from build123d import *

# Parameters (mm, degrees)
EXTRUDE_1_DEPTH = 20
SKETCH_2_R      = 4
EXTRUDE_2_DEPTH = 5
SKETCH_3_W      = 6
SKETCH_3_H      = 6
EXTRUDE_3_DEPTH = 15


with BuildPart() as part:
    # 草图1 → 凸台-拉伸1 (new body)
    with BuildSketch(Plane.XY):
        with BuildLine():
            Line((0, 10), (50, 10))
            ThreePointArc((50, 10), (60, 0), (50, -10))
            Line((50, -10), (0, -10))
            ThreePointArc((0, -10), (-10, 0), (0, 10))
        make_face()
    extrude(amount=EXTRUDE_1_DEPTH)

    # 草图2 → 凸台-拉伸2 (add)
    with BuildSketch(Plane.XY.offset(20)):
        with Locations((50, 0)):
            Circle(SKETCH_2_R)
    extrude(amount=EXTRUDE_2_DEPTH)

    # 草图3 → 凸台-拉伸3 (add)
    with BuildSketch(Plane(origin=(0, 0, 0), x_dir=(-1, 0, 0), z_dir=(0, 0, -1))):
        Rectangle(SKETCH_3_W, SKETCH_3_H)
    extrude(amount=EXTRUDE_3_DEPTH)


solid = part.part
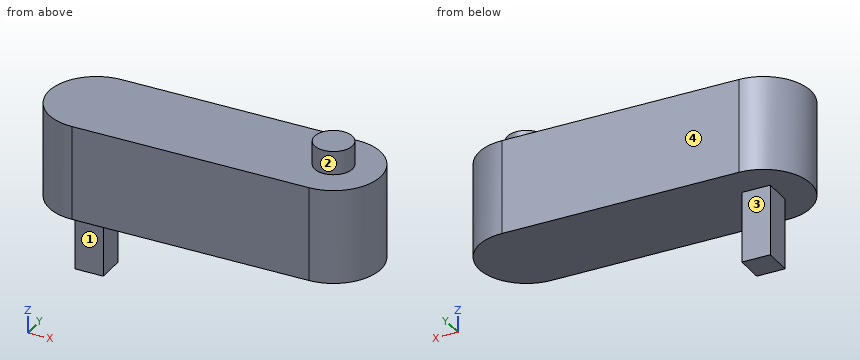
Geometry: final body of the model. Coordinates: model frame, mm. Face numbers are marked on the shaded views. A direction names the side the tool comes from. Round coordinates to 2 decimals unless told otherwise and drop trailing zeros. Loops run counter-clockwise (first coordinate to the right, second up) from the corner with the lowest first, then second, coordinate; pieces in that order, holes last. Notation, with made-up numbers: (80, 47) -> (111, 47) arc R10 cw to (111, 64) -> close; hole circle Ø2 at (6, 3.25). An arc over 180 degrees is marked (long way). One line per question, with ' | ' between items. Start each with the question number.
1. Section D-D on x = 27. Output: boundary loops of the cut face in (y, z).
2. Section B-B on y = 0. Output: boundary loops of the cut face in (x, z), and give its area (3 significant figures).
3. Section A-A on x = 1. Output: boundary loops of the cut face in (y, z), and give its area (3 significant figures).
4. Section C-C on z = 9. Output: boundary loops of the cut face in (x, y).
5. Line query: line 1 along X through (y, z) = (2.25, -5); line 2 along Z through (x, y) = (30.5, 5). Output: solid intervals per line, ascending. Write a range as [from, to].
6. Contact query for flat-ended pins moving along their axis: pin 1 (10 mm diameter, centred on x = 32.5, y = 6.5, fed in from +Z); pin 2 (1.8 mm diameter, centred on x = 1, z = -6.5, fed in from +Y); pin 3 (3 mm diameter, centred on x = -2, z = 3.5, fed in from +Y). Output: stop coordinate, or through.
7. Set-up query: the marked faces 1, 2, 3 and 4. Return all of +Z, -Z, +X, -X, +Y, -Y with unobstructed straight access to the full face (end or side cutting, diameter ignored); none if empty.
Returned:
1) outline: (-10, 0) -> (10, 0) -> (10, 20) -> (-10, 20) -> close
2) outline: (-10, 0) -> (-3, 0) -> (-3, -15) -> (3, -15) -> (3, 0) -> (60, 0) -> (60, 20) -> (54, 20) -> (54, 25) -> (46, 25) -> (46, 20) -> (-10, 20) -> close | area: 1,530 mm2
3) outline: (-10, 0) -> (-3, 0) -> (-3, -15) -> (3, -15) -> (3, 0) -> (10, 0) -> (10, 20) -> (-10, 20) -> close | area: 490 mm2
4) outline: (0, -10) -> (50, -10) arc R10 ccw to (50, 10) -> (0, 10) arc R10 ccw to start
5) line 1: x = [-3, 3] | line 2: z = [0, 20]
6) pin 1: stops at z = 20 | pin 2: stops at y = 3 | pin 3: stops at y = 9.99
7) face 1: -Z, +X, -X, -Y | face 2: +Z | face 3: -Z, +X, -X, +Y | face 4: +Z, -Z, +X, -X, +Y
